```python
from build123d import *

# Parameters (mm, degrees)
SKETCH1_R           = 10
BOSS_EXTRUDE1_DEPTH = 200
CUT_EXTRUDE1_DEPTH  = 201.888028513
BOSS_EXTRUDE2_DEPTH = 7.5
BOSS_EXTRUDE3_DEPTH = 7.5


with BuildPart() as part:
    # Sketch1 → Boss-Extrude1 (new body)
    with BuildSketch(Plane.XY):
        Circle(SKETCH1_R)
    extrude(amount=BOSS_EXTRUDE1_DEPTH)

    # Sketch2 → Cut-Extrude1 (cut, through all)
    with BuildSketch(Plane(origin=(0, 6, 0), x_dir=(1, 0, 0), z_dir=(0, 1, 0))):
        with BuildLine():
            Line((4, -7.366085137), (4, -27.366085137))
            ThreePointArc((4, -27.366085137), (0, -31.366085137), (-4, -27.366085137))
            Line((-4, -27.366085137), (-4, -7.366085137))
            ThreePointArc((-4, -7.366085137), (0, -3.366085137), (4, -7.366085137))
        make_face()
    extrude(amount=CUT_EXTRUDE1_DEPTH, mode=Mode.SUBTRACT)

    # Sketch3 → Boss-Extrude2 (add, symmetric)
    with BuildSketch(Plane.XY.offset(140)):
        with BuildLine():
            ThreePointArc((-4.952730673, 10.930254292), (-10.854939686, -5.115690024), (5.277504453, -10.777195681))
            ThreePointArc((5.277504453, -10.777195681), (10.675038927, -7.586922797), (15.50773958, -3.59239856))
            ThreePointArc((15.50773958, -3.59239856), (16.896032107, -1.149665837), (16.74776808, 1.656099135))
            ThreePointArc((16.74776808, 1.656099135), (7.938689804, 11.069291645), (-4.952730673, 10.930254292))
        make_face()
    extrude(amount=BOSS_EXTRUDE2_DEPTH, both=True)

    # Sketch4 → Boss-Extrude3 (add, symmetric)
    with BuildSketch(Plane.XY.offset(110)):
        with BuildLine():
            ThreePointArc((10.930254292, 4.952730673), (-5.115690024, 10.854939686), (-10.777195681, -5.277504453))
            ThreePointArc((-10.777195681, -5.277504453), (-7.586922797, -10.675038927), (-3.59239856, -15.50773958))
            ThreePointArc((-3.59239856, -15.50773958), (-1.149665837, -16.896032107), (1.656099135, -16.74776808))
            ThreePointArc((1.656099135, -16.74776808), (11.069291645, -7.938689804), (10.930254292, 4.952730673))
        make_face()
    extrude(amount=BOSS_EXTRUDE3_DEPTH, both=True)


solid = part.part
```
Design review of the part built by this model. Coordinates are the model's own, in mm. A direction names the side the tool comes from. Give positions to 0.01 mm unless a question says otherwise; leave off trailing zeros. Write each loop counter-clockwise with the first axis right and the second up, starting at its lowest first coordinate (ties: lowest second). Pieces come first, ordered by that corner, then holes. Notation, with made-up numbers: (48, 7.25) -> (104, 7.25) arc R18 ccw to (104, 25.25) -> close; hole circle Ø8 at (2.25, -24). An arc over 180 degrees is marked (long way). Answer in a Markdown table with one row per item.
(1) Consider section D-D (z = 181). State the section outline as (x, y) points.
Results:
| item | result |
|---|---|
| outline | circle Ø20 at (0, 0) |
(2) Consider section B-B (z = 135.5). State the section outline as (x, y) points, then the cut area to 3 significant figures.
Results:
| item | result |
|---|---|
| outline | (-4.95, 10.93) arc R12 ccw (long way) to (5.28, -10.78) arc R40 ccw to (15.51, -3.59) arc R5 ccw to (16.75, 1.66) arc R16 ccw to start |
| area | 533 mm2 |
(3) Clearance check with flat-ended pins moving along their axes: pin 1 (1.5 mm diameter, centred on y = 6, z = 159, fed in from -X); pin 2 (5 mm diameter, centred on y = 2, z = 65, fed in from +X); pin 3 (3.5 mm diameter, centred on y = 7, z = 21, fed in from +X); pin 4 (12 mm diameter, centred on x = 3.5, y = -10.5, fed in from +Z). State where each tip first meets the part, or that it passes through.
Results:
| item | result |
|---|---|
| pin 1 | x = -8.51 |
| pin 2 | x = 10 |
| pin 3 | x = 8.51 |
| pin 4 | z = 200 |
(4) Consider section A-A (y = 0). State the section outline as (x, z) points.
Results:
| item | result |
|---|---|
| outline | (-12, 102.5) -> (-10, 102.5) -> (-10, 0) -> (10, 0) -> (10, 102.5) -> (12.27, 102.5) -> (12.27, 117.5) -> (10, 117.5) -> (10, 132.5) -> (17.03, 132.5) -> (17.03, 147.5) -> (10, 147.5) -> (10, 200) -> (-10, 200) -> (-10, 147.5) -> (-12, 147.5) -> (-12, 132.5) -> (-10, 132.5) -> (-10, 117.5) -> (-12, 117.5) -> close |
(5) To check wall thickness, follow probe 1 along Z at (x, y) = (3.25, 9.5); probe 2 along Z at (x, y) = (-7, -11.25); probe 3 along X at (y, z) = (0, 159). State the ranges of each line that lie inside material, in increasing order.
Results:
| item | result |
|---|---|
| probe 1 | 102.5 to 117.5, 132.5 to 147.5 |
| probe 2 | 102.5 to 117.5 |
| probe 3 | -10 to 10 |
(6) Mouldability with a two-part tool opening along X and no side actions: class faces 4 (the flat face through (0, 0, 200)), 5 (the cylindrical face through (0.088, 7.974, 31.365)), 6 (the cylindrical face through (11, -8.1, 110.1)) as +X half, -X half, draft (parallel to the pull), parting line (faces both ways), or undercut.
Results:
| item | result |
|---|---|
| face 4 | draft |
| face 5 | undercut |
| face 6 | +X half |
(7) For faces 1 (the cylindrical face through (-2.17, -9.76, 124.9)), 2 (the flat face through (10, 2, 147.5)), 3 (the cylindrical face through (-2.17, -9.76, 50.53)), list the 3-axis set-ups (+Z, -Z, +X, -X, +Y, -Y) from which the entire face can be reached by the end or side of a thin tool; tool diameter is ignored.
Results:
| item | result |
|---|---|
| face 1 | none |
| face 2 | +Z |
| face 3 | -Z |
(8) Consider section C-C (x = 0). State the section outline as (y, z) points, then the cut area to 3 significant figures.
Results:
| item | result |
|---|---|
| outline | (-17.03, 102.5) -> (-10, 102.5) -> (-10, 0) -> (10, 0) -> (10, 3.37) -> (6, 3.37) -> (6, 31.37) -> (10, 31.37) -> (10, 102.5) -> (12, 102.5) -> (12, 117.5) -> (10, 117.5) -> (10, 132.5) -> (12.27, 132.5) -> (12.27, 147.5) -> (10, 147.5) -> (10, 200) -> (-10, 200) -> (-10, 147.5) -> (-12, 147.5) -> (-12, 132.5) -> (-10, 132.5) -> (-10, 117.5) -> (-17.03, 117.5) -> close |
| area | 4,090 mm2 |
